from build123d import *

# Parameters (mm, degrees)
SKETCH1_R           = 0.505
BOSS_EXTRUDE1_DEPTH = 25
SKETCH2_R           = 0.36
BOSS_EXTRUDE2_DEPTH = 6.3
SKETCH3_R           = 0.505
BOSS_EXTRUDE3_DEPTH = 1.4


with BuildPart() as part:
    # Sketch1 → Boss-Extrude1 (new body)
    with BuildSketch(Plane(origin=(0, 0, 0), x_dir=(1, 0, 0), z_dir=(0, 1, 0))):
        with Locations(Location((0, 0, 0), (0, 0, 270))):
            Circle(SKETCH1_R)
    extrude(amount=BOSS_EXTRUDE1_DEPTH)

    # Sketch2 → Boss-Extrude2 (add)
    with BuildSketch(Plane(origin=(0, 25, 0), x_dir=(1, 0, 0), z_dir=(0, 1, 0))):
        with Locations(Location((0, 0, 0), (0, 0, 270))):
            Circle(SKETCH2_R)
    extrude(amount=BOSS_EXTRUDE2_DEPTH)

    # Sketch3 → Boss-Extrude3 (add)
    with BuildSketch(Plane(origin=(0, 31.3, 0), x_dir=(1, 0, 0), z_dir=(0, 1, 0))):
        with Locations(Location((0, 0, 0), (0, 0, 270))):
            Circle(SKETCH3_R)
    extrude(amount=BOSS_EXTRUDE3_DEPTH)

    # Sketch4 → Revolve1 (revolve)
    with BuildSketch(Plane.XY, mode=Mode.PRIVATE) as revolve1_sk:
        Polygon((0, 32.7), (0, 33.2), (0.505, 32.7), align=None)
    revolve(revolve1_sk.sketch.rotate(Axis((0, 32.7, 0), (0, 1, 0)), 90), axis=Axis((0, 32.7, 0), (0, 1, 0)))


solid = part.part
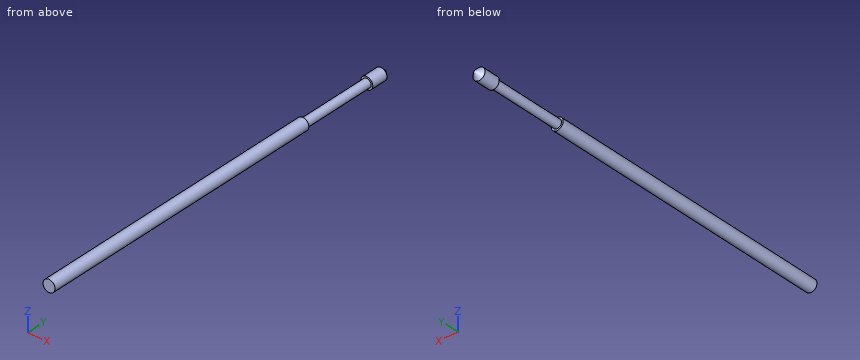
Model file for the job. Use its own axes, mm. Give positions to 0.01 mm unless a question says otherwise; leave off trailing zeros. Write each loop counter-clockwise with the first axis right and the second up, starting at its lowest first coordinate (ties: lowest second). Pieces come first, ordered by that corner, then holes. Notation, with made-up numbers: (42.5, 10) - (54.5, 10) arc R19 cw to (54.5, 24) - close; hole circle Ø11 at (-20.5, -24.75). An arc over 180 degrees is marked (long way). Answer as CSV lines item,"result".
1. Band-saw the part on B-B (y = 24). Write the cut outline in (x, z) (3 decimals), and give its area (3 significant figures).
Responses:
outline,"circle Ø1.01 at (0, 0)"
area,"0.801 mm2"
2. Pin check, flat tip, straight feed: pin 1 (0.5 mm diameter, centred on x = 0, z = 0, fed in from -Y). Stop position of the tip, or through.
Responses:
pin 1,"stops at y = 0"
3. Drill centre lines: L1, parallel to Y at x = 0, z = 0.45; L2, parallel to Z at x = 0.05, y = 11; L3, parallel to X at y = 21, z = 0.4. Where is each one in solid material? Low to high. Write a range as [from, to].
Responses:
L1,"y = [0, 25], [31.3, 32.75]"
L2,"z = [-0.5, 0.5]"
L3,"x = [-0.31, 0.31]"
4. Band-saw the part on A-A (y = 30). Write the cut outline in (x, z).
Responses:
outline,"circle Ø0.72 at (0, 0)"
